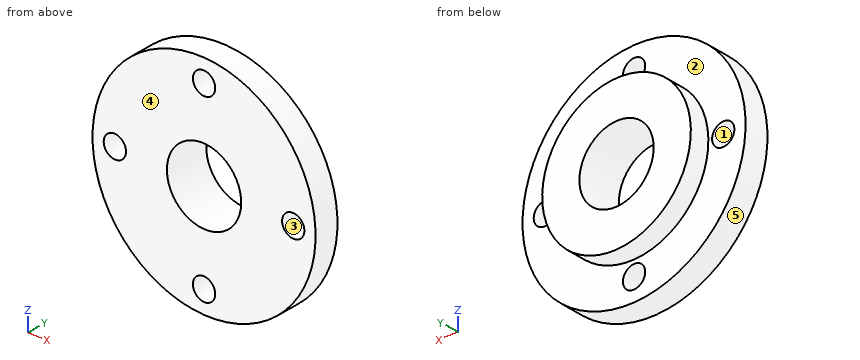
from build123d import *

# Parameters (mm, degrees)
SKETCH_2_R          = 4.5
CUT_EXTRUDE_1_DEPTH = 67.136223055


with BuildPart() as part:
    # 草图1 → 旋转1 (revolve)
    with BuildSketch(Plane.XY, mode=Mode.PRIVATE) as revolve_1_sk:
        Polygon((15, 0), (45, 0), (45, 10), (30, 10), (30, 18), (15, 18), align=None)
    revolve(revolve_1_sk.sketch.rotate(Axis((0, -10, 0), (0, 1, 0)), 90), axis=Axis((0, -10, 0), (0, 1, 0)))

    # 草图2 → 切除-拉伸1 (cut, through all)
    with BuildSketch(Plane(origin=(0, 0, 0), x_dir=(1, 0, 0), z_dir=(0, 1, 0))):
        with Locations(Location((36, 0, 0), (0, 0, 270))):
            Circle(SKETCH_2_R)
        with Locations(Location((0, 36, 0), (0, 0, 270))):
            Circle(SKETCH_2_R)
        with Locations(Location((-36, 0, 0), (0, 0, 270))):
            Circle(SKETCH_2_R)
        with Locations(Location((0, -36, 0), (0, 0, 270))):
            Circle(SKETCH_2_R)
    extrude(amount=CUT_EXTRUDE_1_DEPTH, mode=Mode.SUBTRACT)


solid = part.part
Source: CAD feature listing. Evaluate the final solid. Frame: model axes, mm. Face numbers are marked on the shaded views. A direction names the side the tool comes from. Round coordinates to 2 decimals unless told otherwise and drop trailing zeros. Order: outer loops, then holes, each group sorted by start corner. A loop starts at its lowest first (then second) coordinate and runs counter-clockwise, first axis right, second up. Notation, with made-up numbers: (-17.75, 34.5) - (17.25, 34.5) arc R22 cw to (17.25, 73.5) - close; hole circle Ø3 at (-34, 19.25). An arc over 180 degrees is marked (long way). Use a Markdown table: item, result. Add a question column.
1. Section query A-A (x = 0). Return the cut outline in (y, z).
2. Section query D-D (x = -36). Return the cut outline in (y, z).
3. First-contact query: pin 1 (2 mm diameter, centred on x = 32.5, y = 12, fed in from -Z); pin 2 (8 mm diameter, centred on y = 10.5, z = -33, fed in from -X); pin 3 (6 mm diameter, centred on y = 4.5, z = -4.5, fed in from -X) (3 decimals); pin 4 (11.5 mm diameter, centred on x = 36, z = 0, fed in from +Y). Flat tips, straight axial feed; report the tip coordinate or a pass-through.
4. Section query C-C (z = 36). Return the cut outline in (x, y), then the cut area to 3 significant figures.
5. Mould query, pull axis Z, two halves, no side actions, for the marked faces 3, 4 and 5. Classes: +Z half, -Z half, draft (parallel to the pull), parting line (faces both ways), or undercut.
6. Line query: probe 1 along X at (y, z) = (9.25, 0); probe 2 along Z at (x, y) = (0.5, 7); probe 3 along Y at (x, z) = (-16, -39.5). Output: solid intervals per line, ascending.
7. Section query B-B (z = 0). Return the cut outline in (x, y), then the cut area to 3 significant figures.
8. Set-up query: the marked faces 1 and 2. Return all of +Z, -Z, +X, -X, +Y, -Y with unobstructed straight access to the full face (end or side cutting, diameter ignored); none if empty.
Derived:
| question | item | result |
|---|---|---|
| 1 | outline | (0, -45) - (10, -45) - (10, -40.5) - (0, -40.5) - close; (0, -31.5) - (10, -31.5) - (10, -30) - (18, -30) - (18, -15) - (0, -15) - close; (0, 15) - (18, 15) - (18, 30) - (10, 30) - (10, 31.5) - (0, 31.5) - close; (0, 40.5) - (10, 40.5) - (10, 45) - (0, 45) - close |
| 2 | outline | (0, -27) - (10, -27) - (10, -4.5) - (0, -4.5) - close; (0, 4.5) - (10, 4.5) - (10, 27) - (0, 27) - close |
| 3 | pin 1 | through |
| 3 | pin 2 | x = -34.38 |
| 3 | pin 3 | x = -44.975 |
| 3 | pin 4 | y = 10 |
| 4 | outline | (-27, 0) - (-4.5, 0) - (-4.5, 10) - (-27, 10) - close; (4.5, 0) - (27, 0) - (27, 10) - (4.5, 10) - close |
| 4 | area | 450 mm2 |
| 5 | face 3 | undercut |
| 5 | face 4 | draft |
| 5 | face 5 | parting line |
| 6 | probe 1 | -45 to -40.5, -31.5 to -15, 15 to 31.5, 40.5 to 45 |
| 6 | probe 2 | -45 to -40.47, -31.53 to -14.99, 14.99 to 31.53, 40.47 to 45 |
| 6 | probe 3 | 0 to 10 |
| 7 | outline | (-45, 0) - (-40.5, 0) - (-40.5, 10) - (-45, 10) - close; (-31.5, 0) - (-15, 0) - (-15, 18) - (-30, 18) - (-30, 10) - (-31.5, 10) - close; (15, 0) - (31.5, 0) - (31.5, 10) - (30, 10) - (30, 18) - (15, 18) - close; (40.5, 0) - (45, 0) - (45, 10) - (40.5, 10) - close |
| 7 | area | 660 mm2 |
| 8 | face 1 | +Y, -Y |
| 8 | face 2 | +Y |
